Autodesk Inventor part; units mm, degrees
ref_plane "Work Plane2" through (-7.5, 0, 0) normal (1, 0, 0) x (0, 1, 0)
ref_plane "XZ Plane" through (0, 0, 0) normal (0, 1, 0) x (-1, 0, 0)
ref_plane "XY Plane" through (0, 0, 0) normal (0, 0, 1) x (1, 0, 0)
sketch "Sketch1" plane through (0, 0, 0) normal (1, 0, 0) x (0, 1, 0)
  circle A0 centre (0, 0) radius 4.5
  dimension "d0" = 9
extrude "Extrusion1" add sketch "Sketch1" along normal mid plane 42
sketch "Sketch2" plane through (21, 0, 0) normal (1, 0, 0) x (0, 0, -1)
  circle A0 centre (0, 0) radius 4.5
hole "Hole1" at (21, 0, 0) direction (-1, 0, 0) diameter 5 depth 7 tip angle 118
mirror "Mirror1" about plane through (0, 0, 0) normal (1, 0, 0) of "Hole1"
ref_plane "Work Plane2" through (-7.5, 0, 0) normal (1, 0, 0) x (0, 1, 0)
sketch "Sketch3" plane through (-7.5, 0, 0) normal (1, 0, 0) x (0, 1, 0)
  circle A0 centre (0, 0) radius 15
  dimension "d10" = 30
extrude "Extrusion2" add sketch "Sketch3" along normal blind 4.5
sketch "Sketch4" plane through (-7.5, 0, 0) normal (-1, 0, 0) x (0, 0, 1)
  circle A0 centre (0, 0) radius 10.5
  dimension "d13" = 21
extrude "Extrusion3" add sketch "Sketch4" against normal blind 15
properties part number "dfifferential"
Can you work these out from the model? Positions are in its coordinate system, mm. A direction names the side the tool comes from. Coordinates: 2 decimals unless noted, no trailing zeros. Order: outer loops, then holes, each group sorted by start corner. A loop starts at its lowest first (then second) coordinate and runs counter-clockwise, first axis right, second up. Notation, with made-up numbers: M -39.5,0 L -0.5,0 A25 cw -0.5,20 Z; hole C 36,58 d11. An arc over 180 degrees is marked long. Answer as CSV lines item,"result".
(1) Please list where these lines run through material, in increasing order: L1, parallel to Z at x = -18.5, y = 0; L2, parallel to X at y = 5.5, z = -4.75; L3, parallel to X at y = -4.75, z = -11.
Geometry check:
L1,"-4.5 to -2.5, 2.5 to 4.5"
L2,"-7.5 to 7.5"
L3,"-7.5 to -3"
(2) Suppose I cut it at D-D on x = -9. Please give me the cut outline in (y, z), plus the area to 3 significant figures.
Geometry check:
outline,"C 0,0 d9"
area,"63.6 mm^2"
(3) Suppose I cut it at B-B on z = -3.5. Please give me the cut outline in (x, y), plus the area to 3 significant figures.
Geometry check:
outline,"M -21,-2.83 L -7.5,-2.83 L -7.5,-14.59 L -3,-14.59 L -3,-9.9 L 7.5,-9.9 L 7.5,-2.83 L 21,-2.83 L 21,2.83 L 7.5,2.83 L 7.5,9.9 L -3,9.9 L -3,14.59 L -7.5,14.59 L -7.5,2.83 L -21,2.83 Z"
area,"492 mm^2"
(4) If we mould it in two halves opening along Y, with no side actions, what happens to faces 1 (the cylindrical face through (17.45, 2.44, 0.54)), 2 (the cylindrical face through (2.2, 3.2, 10)), 3 (the flat face through (21, 2, -2))? For each: released by +Y, released by -Y, zero draft, split by the parting line, or undercut.
Geometry check:
face 1,"undercut"
face 2,"split by the parting line"
face 3,"zero draft"
(5) Suppose I cut it at A-A on x = -15. Please give me the cut outline in (y, z).
Geometry check:
outline,"C 0,0 d9; hole C 0,0 d5"
(6) On a 3-axis mill with a long thin cutter (end or side, diameter ignored), from which of +Z, -Z, +X, -X, +Y, -Y can I reach the whole of each face in a straight line? I mean faces 4 (the flat face through (-3, 3.1, 10.2)), 5 (the cylindrical face through (-17.45, -2.44, 0.54)), 6 (the cylindrical face through (-5.281, -14.985, -0.66)). Say none if no direction works.
Geometry check:
face 4,"+X"
face 5,"-X"
face 6,"+X, -X"
(7) Suppose I cut it at C-C on y = 6. Please give me the cut outline in (x, z), plus the area to 3 significant figures.
Geometry check:
outline,"M -7.5,-13.75 L -3,-13.75 L -3,-8.62 L 7.5,-8.62 L 7.5,8.62 L -3,8.62 L -3,13.75 L -7.5,13.75 Z"
area,"305 mm^2"
(8) I'm going to push flat-ended pins straight in: pin 1 (8 mm diameter, centred on y = 0, z = 0, fed in from +X); pin 2 (3 mm diameter, centred on y = -7, z = -8.5, fed in from +X); pin 3 (8 mm diameter, centred on x = 3.5, y = 8.5, fed in from +Z); pin 4 (12 mm diameter, centred on x = 13, y = 0, fed in from -Z). Where does each tip first touch, or does it pass through?
Geometry check:
pin 1,"x = 21"
pin 2,"x = 7.5"
pin 3,"z = 9.49"
pin 4,"z = -10.5"
